```python
from build123d import *

# Parameters (mm, degrees)
F0_R     = 9.525
F1_DEPTH = 63.5
F2_R     = 2.413
F3_R     = 2.413


with BuildPart() as f1:
    # F0 (on Front) → F1 (new body, symmetric)
    with BuildSketch(Plane.XZ):
        Circle(F0_R)
    extrude(amount=F1_DEPTH, both=True)

    # F2
    f2_edges = [f1.edges().sort_by_distance(p)[0] for p in [
        (-9.525, -63.5, 0),
    ]]
    fillet(f2_edges, radius=F2_R)

    # F3
    f3_edges = [f1.edges().sort_by_distance(p)[0] for p in [
        (-9.525, 63.5, 0),
    ]]
    fillet(f3_edges, radius=F3_R)


solid = f1.part
```
Geometry: final body of the model. Coordinates: model frame, mm. Round coordinates to 2 decimals unless told otherwise and drop trailing zeros. Order: outer loops, then holes, each group sorted by start corner. A loop starts at its lowest first (then second) coordinate and runs counter-clockwise, first axis right, second up. Notation, with made-up numbers: (7, 14) -> (27, 14) arc R23 cw to (27, 39) -> close; hole circle Ø10 at (-31.5, 56.25). An arc over 180 degrees is marked (long way). Use CSV: the item, a comma, the result in double quotes. Start each with the question number.
1) First-contact query: pin 1 Ø1.5 at (y, z) = (12.5, -2) entering from -X; pin 2 Ø6 at (x, y) = (3, -32) entering from +Z (3 decimals); pin 3 Ø4 at (x, y) = (5, 38) entering from -Z; pin 4 Ø5 at (y, z) = (-6, 4) entering from +X. Flat tips, straight axial feed; report the tip coordinate or a pass-through.
2) Section A-A (y = 7). Return the cut outline in (x, z) (3 decimals), and give its area (3 significant figures).
3) Material intervals for line 1 along Y through (x, z) = (5.25, 5); line 2 along X through (y, z) = (-1, 3.25); line 3 along X through (y, z) = (-10, -5.5), sorted ascending. Write a range as from..to.
Returned:
1,pin 1,"stops at x = -9.44"
1,pin 2,"stops at z = 9.525"
1,pin 3,"stops at z = -9.04"
1,pin 4,"stops at x = 9.41"
2,outline,"circle Ø19.05 at (0, 0)"
2,area,"285 mm²"
3,line 1,"y = -63.5..63.5"
3,line 2,"x = -8.95..8.95"
3,line 3,"x = -7.78..7.78"
